```python
from build123d import *

# Parameters (mm, degrees)
SKETCH1_R           = 46.6725
BOSS_EXTRUDE1_DEPTH = 4.5
BOSS_EXTRUDE2_START = -4.5
BOSS_EXTRUDE2_DEPTH = 25.4
SKETCH4_R           = 11.9975
SKETCH4_R_2         = 8.8225
BOSS_EXTRUDE3_DEPTH = 3.175


with BuildPart() as part:
    # Sketch1 → Boss-Extrude1 (new body)
    with BuildSketch(Plane.XY):
        Circle(SKETCH1_R)
        with BuildLine():
            Line((-2.927883194, 8.3225), (2.927883194, 8.3225))
            ThreePointArc((2.927883194, 8.3225), (0, -8.8225), (-2.927883194, 8.3225))
        make_face(mode=Mode.SUBTRACT)
    extrude(amount=BOSS_EXTRUDE1_DEPTH)

    # Sketch2 → Boss-Extrude2 (add)
    with BuildSketch(Plane.XY.offset(4.5).offset(BOSS_EXTRUDE2_START)):
        with BuildLine():
            Line((-2.25, 46.618234161), (-2.25, 13.778350254))
            ThreePointArc((-2.25, 13.778350254), (-3.318707206, 12.385583908), (-4.940617969, 13.057401343))
            Line((-4.940617969, 13.057401343), (-21.360559922, 41.497575063))
            ThreePointArc((-21.360559922, 41.497575063), (-23.33625, 40.419570658), (-25.257674239, 39.247575063))
            Line((-25.257674239, 39.247575063), (-8.837732286, 10.807401343))
            ThreePointArc((-8.837732286, 10.807401343), (-9.066876702, 9.066876702), (-10.807401343, 8.837732286))
            Line((-10.807401343, 8.837732286), (-39.247575063, 25.257674239))
            ThreePointArc((-39.247575063, 25.257674239), (-40.419570658, 23.33625), (-41.497575063, 21.360559922))
            Line((-41.497575063, 21.360559922), (-13.057401343, 4.940617969))
            ThreePointArc((-13.057401343, 4.940617969), (-12.385583908, 3.318707206), (-13.778350254, 2.25))
            Line((-13.778350254, 2.25), (-46.618234161, 2.25))
            ThreePointArc((-46.618234161, 2.25), (-46.6725, 0), (-46.618234161, -2.25))
            Line((-46.618234161, -2.25), (-13.778350254, -2.25))
            ThreePointArc((-13.778350254, -2.25), (-12.385583908, -3.318707206), (-13.057401343, -4.940617969))
            Line((-13.057401343, -4.940617969), (-41.497575063, -21.360559922))
            ThreePointArc((-41.497575063, -21.360559922), (-40.419570658, -23.33625), (-39.247575063, -25.257674239))
            Line((-39.247575063, -25.257674239), (-10.807401343, -8.837732286))
            ThreePointArc((-10.807401343, -8.837732286), (-9.066876702, -9.066876702), (-8.837732286, -10.807401343))
            Line((-8.837732286, -10.807401343), (-25.257674239, -39.247575063))
            ThreePointArc((-25.257674239, -39.247575063), (-23.33625, -40.419570658), (-21.360559922, -41.497575063))
            Line((-21.360559922, -41.497575063), (-4.940617969, -13.057401343))
            ThreePointArc((-4.940617969, -13.057401343), (-3.318707206, -12.385583908), (-2.25, -13.778350254))
            Line((-2.25, -13.778350254), (-2.25, -46.618234161))
            ThreePointArc((-2.25, -46.618234161), (0, -46.6725), (2.25, -46.618234161))
            Line((2.25, -46.618234161), (2.25, -13.778350254))
            ThreePointArc((2.25, -13.778350254), (3.318707206, -12.385583908), (4.940617969, -13.057401343))
            Line((4.940617969, -13.057401343), (21.360559922, -41.497575063))
            ThreePointArc((21.360559922, -41.497575063), (23.33625, -40.419570658), (25.257674239, -39.247575063))
            Line((25.257674239, -39.247575063), (8.837732286, -10.807401343))
            ThreePointArc((8.837732286, -10.807401343), (9.066876702, -9.066876702), (10.807401343, -8.837732286))
            Line((10.807401343, -8.837732286), (39.247575063, -25.257674239))
            ThreePointArc((39.247575063, -25.257674239), (40.419570658, -23.33625), (41.497575063, -21.360559922))
            Line((41.497575063, -21.360559922), (13.057401343, -4.940617969))
            ThreePointArc((13.057401343, -4.940617969), (12.385583908, -3.318707206), (13.778350254, -2.25))
            Line((13.778350254, -2.25), (46.618234161, -2.25))
            ThreePointArc((46.618234161, -2.25), (46.6725, 0), (46.618234161, 2.25))
            Line((46.618234161, 2.25), (13.778350254, 2.25))
            ThreePointArc((13.778350254, 2.25), (12.385583908, 3.318707206), (13.057401343, 4.940617969))
            Line((13.057401343, 4.940617969), (41.497575063, 21.360559922))
            ThreePointArc((41.497575063, 21.360559922), (40.419570658, 23.33625), (39.247575063, 25.257674239))
            Line((39.247575063, 25.257674239), (10.807401343, 8.837732286))
            ThreePointArc((10.807401343, 8.837732286), (9.066876702, 9.066876702), (8.837732286, 10.807401343))
            Line((8.837732286, 10.807401343), (25.257674239, 39.247575063))
            ThreePointArc((25.257674239, 39.247575063), (23.33625, 40.419570658), (21.360559922, 41.497575063))
            Line((21.360559922, 41.497575063), (4.940617969, 13.057401343))
            ThreePointArc((4.940617969, 13.057401343), (3.318707206, 12.385583908), (2.25, 13.778350254))
            Line((2.25, 13.778350254), (2.25, 46.618234161))
            ThreePointArc((2.25, 46.618234161), (0, 46.6725), (-2.25, 46.618234161))
        make_face()
        with BuildLine():
            Line((2.927883194, 8.3225), (-2.927883194, 8.3225))
            ThreePointArc((-2.927883194, 8.3225), (0, -8.8225), (2.927883194, 8.3225))
        make_face(mode=Mode.SUBTRACT)
    extrude(amount=BOSS_EXTRUDE2_DEPTH)

    # Sketch3 → Cut-Revolve1 (revolve, cut)
    with BuildSketch(Plane(origin=(0, 0, 0), x_dir=(1, 0, 0), z_dir=(0, 1, 0)), mode=Mode.PRIVATE) as cut_revolve1_sk:
        Polygon((-24.13, -12.7), (-6.35, -12.7), (-6.35, -25.4), (-35.56, -25.4), align=None)
    revolve(cut_revolve1_sk.sketch.rotate(Axis((0, 0, 0), (0, 0, 1)), 2.76320082), axis=Axis((0, 0, 0), (0, 0, 1)), mode=Mode.SUBTRACT)

    # Sketch4 → Boss-Extrude3 (add)
    with BuildSketch(Plane.XY.offset(12.7)):
        with Locations(Location((0, 0, 0), (0, 0, 180))):
            Circle(SKETCH4_R)
        with Locations(Location((0, 0, 0), (0, 0, 109.382041685))):
            Circle(SKETCH4_R_2, mode=Mode.SUBTRACT)
    extrude(amount=BOSS_EXTRUDE3_DEPTH)


solid = part.part
```
Part model, mm, in its own coordinate system. A direction names the side the tool comes from. Round coordinates to 2 decimals unless told otherwise and drop trailing zeros. Loops run counter-clockwise (first coordinate to the right, second up) from the corner with the lowest first, then second, coordinate; pieces in that order, holes last. Notation, with made-up numbers: (23.5, -10) -> (74.5, -10) arc R29 cw to (74.5, 10) -> close; hole circle Ø7 at (75, 21). An arc over 180 degrees is marked (long way). Use one line per item in the form item = value. Start each with the question number.
Item 1: Two-plate mould, pull along X, no slides. Class faces 4 (the cylindrical face through (12.38, -3.34, 8.54)), 5 (the flat face through (-30.24, -14.86, 12.48)), 6 (the cylindrical face through (8.84, -8.11, 14.27)), 7 (the flat face through (34, -2.25, 12)): released by +X, released by -X, zero draft, split by the parting line, or undercut.
Item 2: Drop flat-ended pins along their axis: pin 1 Ø6 at (x, z) = (-33, 7) entering from +Y; pin 2 Ø9.5 at (x, y) = (-13.5, -26) entering from +Z; pin 3 Ø12 at (y, z) = (-32.5, 18.5) entering from -X; pin 4 Ø7 at (x, y) = (-2, 3.5) entering from +Z. Give the stop position or say it passes through.
Item 3: Band-saw the part on B-B (x = 0). List the corners of the cut face in (y, z) (1 decimal), plus the area to 3 significant figures.
Item 4: Band-saw the part on C-C (z = 20.75). Give the number of separate pieces and of enclosed holes in the cut face, plus the area to 3 significant figures.
Item 5: Band-saw the part on A-A (y = 0). List the corners of the cut face in (x, z) (1 decimal), plus the area to 3 significant figures.
Item 6: Drill centre lines: line 1 along X through (y, z) = (18.5, 12); line 2 along X through (y, z) = (-31.5, 15.25); line 3 along X through (y, z) = (27, 8). Where is each one in solid material? Low to high.
Item 7: Tool access for faces 1 (the cylindrical face through (-3.293, 12.393, 8.543)), 2 (the flat face through (-28.39, -18.99, 12.48)), 3 (the flat face through (-15.09, -30.64, 12.48)): list every direction of +Z, -Z, +X, -X, +Y, -Y with a clear straight run to the whole face (end or side of a thin tool).
Data:
q1.face_4 = released by +X
q1.face_5 = released by -X
q1.face_6 = undercut
q1.face_7 = zero draft
q2.pin_1 = 34.58
q2.pin_2 = 23.72
q2.pin_3 = -24.83
q2.pin_4 = through
q3.outline = (-46.7, 0) -> (-8.8, 0) -> (-8.8, 15.9) -> (-12, 15.9) -> (-12, 12.7) -> (-24.1, 12.7) -> (-35.6, 25.4) -> (-46.7, 25.4) -> close; (8.3, 0) -> (46.7, 0) -> (46.7, 25.4) -> (35.6, 25.4) -> (24.1, 12.7) -> (12, 12.7) -> (12, 15.9) -> (8.8, 15.9) -> (8.8, 12.7) -> (8.3, 12.7) -> close
q3.area = 1,420 mm^2
q4.separate_pieces = 12
q4.enclosed_holes = 0
q4.area = 827 mm^2
q5.outline = (-46.7, 0) -> (-8.8, 0) -> (-8.8, 15.9) -> (-12, 15.9) -> (-12, 12.7) -> (-24.1, 12.7) -> (-35.6, 25.4) -> (-46.7, 25.4) -> close; (8.8, 0) -> (46.7, 0) -> (46.7, 25.4) -> (35.6, 25.4) -> (24.1, 12.7) -> (12, 12.7) -> (12, 15.9) -> (8.8, 15.9) -> close
q5.area = 1,410 mm^2
q6.line_1 = -36.54 to -27.54, -13.28 to -8.08, -2.25 to 2.25, 8.08 to 13.28, 27.54 to 36.54
q6.line_2 = -20.78 to -15.59, -2.25 to 2.25, 15.59 to 20.78
q6.line_3 = -18.19 to -12.99, -2.25 to 2.25, 12.99 to 18.19
q7.face_1 = +Z, +Y
q7.face_2 = +Z
q7.face_3 = +Z, -Y
